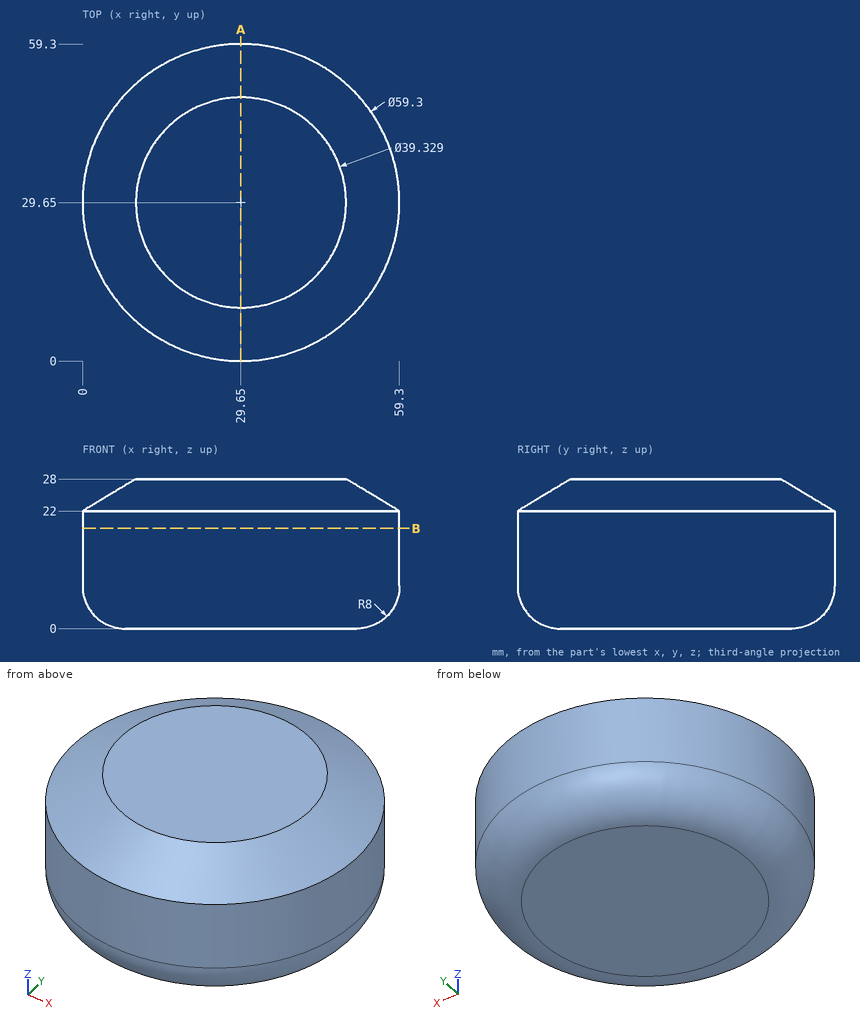
Geometry check sheet. Reference: drawing and pictorial views, mm from the part's lowest x, y, z. Give positions to 0.01 mm unless a question says otherwise; leave off trailing zeros. Order: outer loops, then holes, each group sorted by start corner. A loop starts at its lowest first (then second) coordinate and runs counter-clockwise, first axis right, second up. Notation, with made-up numbers: (-17, 78.5) - (18, 78.5) arc R20 cw to (18, 113.5) - close; hole circle Ø8 at (-15, 45). An arc over 180 degrees is marked (long way). Use one line per item in the form item = value.
1) Sectioned sample at A-A (x = 29.65). Record the boundary of the cut face in (y, z) (1 decimal), and give its area (3 significant figures).
Working result:
outline = (0, 8) arc R8 ccw to (8, 0) - (51.3, 0) arc R8 ccw to (59.3, 8) - (59.3, 22) - (49.3, 28) - (10, 28) - (0, 22) - close
area = 1,570 mm^2
2) Sectioned sample at B-B (z = 18.75). Record the boundary of the cut face in (x, y).
Working result:
outline = circle Ø59.3 at (29.65, 29.65)
3) Material ranges on probe 1 along X at (y, z) = (29.5, 21.75); probe 2 along Z at (x, y) = (50, 43) (1 decimal); probe 3 along X at (y, z) = (30.5, 2.25), recorded low to high. Write a range as from..to.
Working result:
probe_1 = 0..59.3
probe_2 = 0.5..25.2
probe_3 = 2.45..56.85
4) Depth check by flat-ended pin: pin 1 Ø1.5 at (x, z) = (51, 22) entering from +Y (1 decimal); pin 2 Ø8 at (y, z) = (53, 6) entering from -X; pin 3 Ø8 at (x, y) = (50, 35) entering from -Z; pin 4 Ø12 at (x, z) = (49.5, 18.5) entering from -Y. Enter the tip coordinate at first touch or a pass-through.
Working result:
pin_1 = 51
pin_2 = 7.37
pin_3 = 0
pin_4 = 3.43
